from build123d import *

# Parameters (mm, degrees)
CROQUIS1_W              = 350
CROQUIS1_H              = 170
SALIENTE_EXTRUIR1_DEPTH = 6.35
CROQUIS2_W              = 6.35
CROQUIS2_H              = 20
SALIENTE_EXTRUIR2_DEPTH = 6.35
CROQUIS4_W              = 20
CROQUIS4_H              = 6.35
CORTAR_EXTRUIR1_DEPTH   = 10


with BuildPart() as part:
    # Croquis1 → Saliente-Extruir1 (new body)
    with BuildSketch(Plane.XY):
        with Locations((18.650000026, 65)):
            Rectangle(CROQUIS1_W, CROQUIS1_H)
    extrude(amount=SALIENTE_EXTRUIR1_DEPTH)

    # Croquis2 → Saliente-Extruir2 (add)
    with BuildSketch(Plane.ZY.offset(156.349999974)):
        with Locations((3.175, 108)):
            Rectangle(CROQUIS2_W, CROQUIS2_H)
        with Locations((3.175, 22)):
            Rectangle(CROQUIS2_W, CROQUIS2_H)
    saliente_extruir2 = extrude(amount=SALIENTE_EXTRUIR2_DEPTH)

    # Simetría1: Saliente-Extruir2 across plane
    add(saliente_extruir2.mirror(Plane(origin=(18.650000026, 0, 0), x_dir=(0, 0, 1), z_dir=(1, 0, 0))))

    # Croquis4 → Cortar-Extruir1 (cut)
    with BuildSketch(Plane.XY.offset(6.35)):
        with Locations((18.650000026, 11.335)):
            Rectangle(CROQUIS4_W, CROQUIS4_H)
        with Locations((108.650000026, 11.335)):
            Rectangle(CROQUIS4_W, CROQUIS4_H)
        with Locations((-71.349999974, 11.335)):
            Rectangle(CROQUIS4_W, CROQUIS4_H)
    extrude(amount=-CORTAR_EXTRUIR1_DEPTH, mode=Mode.SUBTRACT)


solid = part.part
The listing builds one solid part. Answer for the finished solid, in the listing's coordinates (mm). A direction names the side the tool comes from. Give positions to 0.01 mm unless a question says otherwise; leave off trailing zeros. Loops run counter-clockwise (first coordinate to the right, second up) from the corner with the lowest first, then second, coordinate; pieces in that order, holes last.
Item 1: A tool of negligible diameter and unlimited length cuts with its end or side. For faces 5 (the flat face through (197, 12, 3)), 6 (the flat face through (-159, 12, 3)), 7 (the flat face through (-156.35, 134, 3)), 8 (the flat face through (197, 98, 3)), from which of +Z, -Z, +X, -X, +Y, -Y can it reach the whole face along a straight path? Write none if from no direction.
Derived:
face 5: +Z, -Z, +X, -Y
face 6: +Z, -Z, -X, -Y
face 7: +Z, -Z, -X, +Y
face 8: +Z, -Z, +X
Item 2: Each of these flat-tipped pins is pushed along its axis until it touches: pin 1 Ø1.9 at (y, z) = (11, 3) entering from +X; pin 2 Ø1.9 at (x, z) = (196.5, 3.5) entering from +Y; pin 3 Ø1 at (y, z) = (8.5, 2.5) entering from -X. Where does it stop, or does it pass through?
Derived:
pin 1: stops at x = 193.65
pin 2: stops at y = 118
pin 3: stops at x = -156.35
Item 3: A cutting plane is placed at A-A (z = 5). Give the number of separate pieces and of enclosed holes in the cut face, then the cut area to 3 significant figures.
Derived:
separate pieces: 1
enclosed holes: 3
area: 59,600 mm2
Item 4: Determine the mould class of faces 1 (the flat face through (16, -20, 3)), 2 (the flat face through (98.65, 11, 3)), 3 (the flat face through (16, 66, 0)), 4 (the flat face through (-81.35, 11, 3)) for opening direction Y: +Y half, -Y half, draft (parallel to the pull), parting line (faces both ways), or undercut.
Derived:
face 1: -Y half
face 2: undercut
face 3: draft
face 4: undercut
Item 5: Find the intervals of material crossed by line 1 along Y through (x, z) = (24.5, 2); line 2 along X through (y, z) = (36, 5.75), in increasing order.
Derived:
line 1: y = -20 to 8.16, 14.51 to 150
line 2: x = -156.35 to 193.65
Item 6: A cutting plane is placed at B-B (y = 82). Give the vertices of the cut face in (x, z).
Derived:
outline: (-156.35, 0) - (193.65, 0) - (193.65, 6.35) - (-156.35, 6.35) - close
